from build123d import *

# Parameters (mm, degrees)
SKETCH_1_W          = 90
SKETCH_1_H          = 60
EXTRUDE_1_DEPTH     = 100
SKETCH_2_W          = 10
SKETCH_2_H          = 30
CUT_EXTRUDE_1_DEPTH = 5


with BuildPart() as part:
    # Эскиз1 → Бобышка-Вытянуть1 (new, symmetric)
    with BuildSketch(Plane.XY):
        Rectangle(SKETCH_1_W, SKETCH_1_H)
    extrude(amount=EXTRUDE_1_DEPTH, both=True)

    # Эскиз2 → Вырез-Вытянуть1 (cut)
    with BuildSketch(Plane.XY.offset(100)):
        with Locations((-30, 0)):
            Rectangle(SKETCH_2_W, SKETCH_2_H)
        with Locations((30, 0)):
            Rectangle(SKETCH_2_W, SKETCH_2_H)
    extrude(amount=-CUT_EXTRUDE_1_DEPTH, mode=Mode.SUBTRACT)


solid = part.part
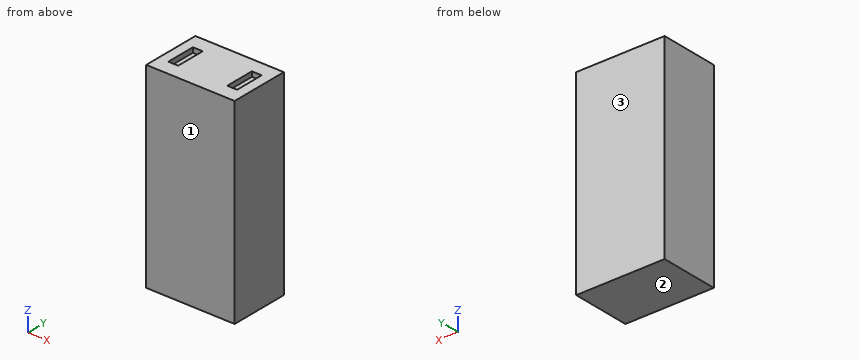
Geometry: final body of the model. Coordinates: model frame, mm. Face numbers are marked on the shaded views. Coordinates: 2 decimals unless noted, no trailing zeros. Return JSON: item names as keys, results as strings.
Item 1: Pin query (flat end, axial travel): pin 1 Ø3 at (x, y) = (-31, 6.5) entering from +Z. Return the tip coordinate at first contact, or that it passes through.
Completed:
{"pin 1": "stops at z = 95"}
Item 2: Pull-direction query (Y, two-part tool) for the marked faces 1, 2 and 3; classes: +Y half, -Y half, draft (parallel to the pull), parting line (faces both ways), or undercut.
Completed:
{"face 1": "-Y half", "face 2": "draft", "face 3": "+Y half"}
Item 3: Line query: L1, parallel to Z at x = 31, y = -3. Output: solid intervals per line, ascending.
Completed:
{"L1": "z = -100 to 95"}
